```python
from build123d import *

# Parameters (mm, degrees)
SKETCH1_R           = 12.09
SKETCH1_R_2         = 1.75
SKETCH1_R_3         = 1.995
BOSS_EXTRUDE1_DEPTH = 4


with BuildPart() as part:
    # Sketch1 → Boss-Extrude1 (new body)
    # profile 1 of 22: a face of its own
    with BuildSketch(Plane.XY):
        Circle(SKETCH1_R)
        Circle(SKETCH1_R_2, mode=Mode.SUBTRACT)
    # profile 2 of 22: a face of its own
    with BuildSketch(Plane.XY):
        with BuildLine():
            ThreePointArc((14.051469909, -4.073462091), (14.048317136, -4.084321933), (14.04515597, -4.095179336))
            Line((14.04515597, -4.095179336), (30.82582707, -3.999919373))
            ThreePointArc((30.82582707, -3.999919373), (34.803112279, -0.008027822), (30.841914591, 3.999828048))
            Line((30.841914591, 3.999828048), (14.04515597, 4.095179336))
            ThreePointArc((14.04515597, 4.095179336), (14.128586435, 3.797360314), (14.205702589, 3.497844187))
            ThreePointArc((14.205702589, 3.497844187), (14.50484412, 1.909554151), (14.626965513, 0.297959519))
            ThreePointArc((14.626965513, 0.297959519), (14.629241359, 0.148987485), (14.63, 0))
            ThreePointArc((14.63, 0), (14.629241116, -0.149011314), (14.626964543, -0.298007168))
            ThreePointArc((14.626964543, -0.298007168), (14.504858624, -1.909443973), (14.20576712, -3.497582099))
            ThreePointArc((14.20576712, -3.497582099), (14.131552306, -3.786308154), (14.051469909, -4.073462091))
        make_face()
        with Locations((30.75, 0)):
            Circle(SKETCH1_R_3, mode=Mode.SUBTRACT)
    # profile 3 of 22: a face of its own
    with BuildSketch(Plane.XY):
        with BuildLine():
            ThreePointArc((14.205702589, 3.497844187), (14.128586435, 3.797360314), (14.04515597, 4.095179336))
            Line((14.04515597, 4.095179336), (13.966164937, 4.095627749))
            Line((13.966164937, 4.095627749), (11.369827915, 4.11036655))
            ThreePointArc((11.369827915, 4.11036655), (11.678097516, 3.128919686), (11.901816808, 2.124819208))
            ThreePointArc((11.901816808, 2.124819208), (13.1403578, 2.666023245), (14.205702589, 3.497844187))
        make_face()
    # profile 4 of 22: a face of its own
    with BuildSketch(Plane.XY):
        with BuildLine():
            ThreePointArc((-12.517636695, -7.572692492), (-11.175984377, -7.407777173), (-9.917325106, -6.914821961))
            ThreePointArc((-9.917325106, -6.914821961), (-10.469253219, -6.046721181), (-10.945386333, -5.134843524))
            ThreePointArc((-10.945386333, -5.134843524), (-12.001489862, -5.978375477), (-12.815033037, -7.057749518))
            ThreePointArc((-12.815033037, -7.057749518), (-12.668951436, -7.31673216), (-12.517636695, -7.572692492))
        make_face()
    # profile 5 of 22: a face of its own
    with BuildSketch(Plane.XY):
        with BuildLine():
            ThreePointArc((-14.051145033, -4.074582586), (-12.712516328, -4.262616236), (-11.369129658, -4.112297512))
            ThreePointArc((-11.369129658, -4.112297512), (-11.677558471, -3.130930876), (-11.901445615, -2.126897335))
            ThreePointArc((-11.901445615, -2.126897335), (-13.139881298, -2.668425004), (-14.205038564, -3.500539874))
            ThreePointArc((-14.205038564, -3.500539874), (-14.13100701, -3.788342761), (-14.051145033, -4.074582586))
        make_face()
    # profile 6 of 22: a face of its own
    with BuildSketch(Plane.XY):
        with BuildLine():
            ThreePointArc((-14.626950262, -0.298707293), (-13.382615157, -0.826868574), (-12.046093246, -1.029435529))
            ThreePointArc((-12.046093246, -1.029435529), (-12.089999882, -0.001686428), (-12.046379968, 1.026074882))
            ThreePointArc((-12.046379968, 1.026074882), (-13.382791491, 0.823465153), (-14.62701917, 0.295313712))
            ThreePointArc((-14.62701917, 0.295313712), (-14.629999902, -0.00169714), (-14.626950262, -0.298707293))
        make_face()
    # profile 7 of 22: a face of its own
    with BuildSketch(Plane.XY):
        with BuildLine():
            ThreePointArc((-14.205774364, 3.497552675), (-13.140565234, 2.66528054), (-11.902026335, 2.123645243))
            ThreePointArc((-11.902026335, 2.123645243), (-11.678416405, 3.127729251), (-11.370260409, 4.109170017))
            ThreePointArc((-11.370260409, 4.109170017), (-12.71360248, 4.259309779), (-14.052145793, 4.071129894))
            ThreePointArc((-14.052145793, 4.071129894), (-14.131870386, 3.78512079), (-14.205774364, 3.497552675))
        make_face()
    # profile 8 of 22: a face of its own
    with BuildSketch(Plane.XY):
        with BuildLine():
            ThreePointArc((-9.919135011, 6.912225448), (-11.177872267, 7.404913556), (-12.519533027, 7.569556974))
            ThreePointArc((-12.519533027, 7.569556974), (-12.670533379, 7.313992337), (-12.816317544, 7.055416686))
            ThreePointArc((-12.816317544, 7.055416686), (-12.00284137, 5.975783406), (-10.94671211, 5.132016561))
            ThreePointArc((-10.94671211, 5.132016561), (-10.470825179, 6.043998682), (-9.919135011, 6.912225448))
        make_face()
    # profile 9 of 22: a face of its own
    with BuildSketch(Plane.XY):
        with BuildLine():
            ThreePointArc((-7.791898403, 9.244155952), (-8.880242473, 10.045843984), (-10.13359017, 10.552120653))
            ThreePointArc((-10.13359017, 10.552120653), (-10.345575707, 10.344368676), (-10.553302948, 10.1323589))
            ThreePointArc((-10.553302948, 10.1323589), (-10.04699158, 8.878969486), (-9.245249077, 7.790601357))
            ThreePointArc((-9.245249077, 7.790601357), (-8.549520677, 8.54832125), (-7.791898403, 9.244155952))
        make_face()
    # profile 10 of 22: a face of its own
    with BuildSketch(Plane.XY):
        with BuildLine():
            ThreePointArc((-5.133551517, 10.945992364), (-5.977311447, 12.002061971), (-7.05691548, 12.815492339))
            ThreePointArc((-7.05691548, 12.815492339), (-7.315469666, 12.669680484), (-7.571012334, 12.518652972))
            ThreePointArc((-7.571012334, 12.518652972), (-7.40634855, 11.176941958), (-6.913615931, 9.918165897))
            ThreePointArc((-6.913615931, 9.918165897), (-6.045466706, 10.469977665), (-5.133551517, 10.945992364))
        make_face()
    # profile 11 of 22: a face of its own
    with BuildSketch(Plane.XY):
        with BuildLine():
            ThreePointArc((-2.125311093, 11.901728982), (-2.666957342, 13.14020836), (-3.499215334, 14.205364904))
            ThreePointArc((-3.499215334, 14.205364904), (-3.786765286, 14.131429817), (-4.072755654, 14.051674682))
            ThreePointArc((-4.072755654, 14.051674682), (-4.260931239, 12.713077321), (-4.110760617, 11.369685446))
            ThreePointArc((-4.110760617, 11.369685446), (-3.129363382, 11.677978627), (-2.125311093, 11.901728982))
        make_face()
    # profile 12 of 22: a face of its own
    with BuildSketch(Plane.XY):
        with BuildLine():
            ThreePointArc((1.027754616, 12.046236775), (0.825159863, 13.382704508), (0.296996585, 14.626985097))
            ThreePointArc((0.296996585, 14.626985097), (0, 14.63), (-0.296996585, 14.626985097))
            ThreePointArc((-0.296996585, 14.626985097), (-0.825159863, 13.382704508), (-1.027754616, 12.046236775))
            ThreePointArc((-1.027754616, 12.046236775), (0, 12.09), (1.027754616, 12.046236775))
        make_face()
    # profile 13 of 22: a face of its own
    with BuildSketch(Plane.XY):
        with BuildLine():
            ThreePointArc((4.110717434, 11.369701059), (4.260994095, 12.713043392), (4.072942889, 14.051620413))
            ThreePointArc((4.072942889, 14.051620413), (3.786710214, 14.131444574), (3.498915331, 14.2054388))
            ThreePointArc((3.498915331, 14.2054388), (2.666773966, 13.14023428), (2.125244746, 11.901740829))
            ThreePointArc((2.125244746, 11.901740829), (3.129308654, 11.677993293), (4.110717434, 11.369701059))
        make_face()
    # profile 14 of 22: a face of its own
    with BuildSketch(Plane.XY):
        with BuildLine():
            ThreePointArc((6.913450185, 9.91828143), (7.406352802, 11.176909529), (7.571236986, 12.518517105))
            ThreePointArc((7.571236986, 12.518517105), (7.315275528, 12.669792577), (7.056292749, 12.81583523))
            ThreePointArc((7.056292749, 12.81583523), (5.976880257, 12.002254067), (5.133331053, 10.946095756))
            ThreePointArc((5.133331053, 10.946095756), (6.045273784, 10.470089058), (6.913450185, 9.91828143))
        make_face()
    # profile 15 of 22: a face of its own
    with BuildSketch(Plane.XY):
        with BuildLine():
            ThreePointArc((9.244954117, 7.790951378), (10.046869152, 8.879052728), (10.553440202, 10.132215942))
            ThreePointArc((10.553440202, 10.132215942), (10.345229175, 10.344715236), (10.132740224, 10.552936821))
            ThreePointArc((10.132740224, 10.552936821), (8.879594749, 10.046380548), (7.791503622, 9.244488699))
            ThreePointArc((7.791503622, 9.244488699), (8.549176321, 8.548665641), (9.244954117, 7.790951378))
        make_face()
    # profile 16 of 22: a face of its own
    with BuildSketch(Plane.XY):
        with BuildLine():
            ThreePointArc((10.946374382, 5.132736881), (12.002615026, 5.976132183), (12.81632055, 7.055411226))
            ThreePointArc((12.81632055, 7.055411226), (12.670115094, 7.314716911), (12.518663963, 7.570994161))
            ThreePointArc((12.518663963, 7.570994161), (11.17714698, 7.405952739), (9.918639175, 6.912936924))
            ThreePointArc((9.918639175, 6.912936924), (10.47040953, 6.044718709), (10.946374382, 5.132736881))
        make_face()
    # profile 17 of 22: a face of its own
    with BuildSketch(Plane.XY):
        with BuildLine():
            ThreePointArc((12.046231207, -1.027819886), (11.986581537, -1.577961676), (11.901820644, -2.124797724))
            ThreePointArc((11.901820644, -2.124797724), (13.140374441, -2.665881604), (14.20576712, -3.497582099))
            ThreePointArc((14.20576712, -3.497582099), (14.504858624, -1.909443973), (14.626964543, -0.298007168))
            ThreePointArc((14.626964543, -0.298007168), (13.382627003, -0.825679814), (12.046231207, -1.027819886))
        make_face()
    # profile 18 of 22: a face of its own
    with BuildSketch(Plane.XY):
        with BuildLine():
            ThreePointArc((11.901820644, -2.124797724), (11.67810034, -3.128909147), (11.369827915, -4.11036655))
            Line((11.369827915, -4.11036655), (13.967019497, -4.095622898))
            ThreePointArc((13.967019497, -4.095622898), (14.009289492, -4.084713176), (14.051469909, -4.073462091))
            ThreePointArc((14.051469909, -4.073462091), (14.131552306, -3.786308154), (14.20576712, -3.497582099))
            ThreePointArc((14.20576712, -3.497582099), (13.140374441, -2.665881604), (11.901820644, -2.124797724))
        make_face()
    # profile 19 of 22: a face of its own
    with BuildSketch(Plane.XY):
        with BuildLine():
            ThreePointArc((12.09, 0), (12.079052845, -0.514375696), (12.046231207, -1.027819886))
            ThreePointArc((12.046231207, -1.027819886), (13.382627003, -0.825679814), (14.626964543, -0.298007168))
            ThreePointArc((14.626964543, -0.298007168), (14.629241116, -0.149011314), (14.63, 0))
            ThreePointArc((14.63, 0), (14.629241359, 0.148987485), (14.626965513, 0.297959519))
            ThreePointArc((14.626965513, 0.297959519), (13.382629481, 0.825632028), (12.046235232, 1.027772701))
            ThreePointArc((12.046235232, 1.027772701), (12.079053853, 0.514352039), (12.09, 0))
        make_face()
    # profile 20 of 22: a face of its own
    with BuildSketch(Plane.XY):
        with BuildLine():
            ThreePointArc((11.901816808, 2.124819208), (11.986583203, 1.577949019), (12.046235232, 1.027772701))
            ThreePointArc((12.046235232, 1.027772701), (13.382629481, 0.825632028), (14.626965513, 0.297959519))
            ThreePointArc((14.626965513, 0.297959519), (14.50484412, 1.909554151), (14.205702589, 3.497844187))
            ThreePointArc((14.205702589, 3.497844187), (13.1403578, 2.666023245), (11.901816808, 2.124819208))
        make_face()
    # profile 21 of 22: a face of its own
    with BuildSketch(Plane.XY):
        with BuildLine():
            Line((11.369827915, 4.11036655), (13.966164937, 4.095627749))
            ThreePointArc((13.966164937, 4.095627749), (12.668895431, 4.261362771), (11.369827915, 4.11036655))
        make_face()
    # profile 22 of 22: a face of its own
    with BuildSketch(Plane.XY):
        with BuildLine():
            ThreePointArc((-10.130994605, -10.554612656), (-8.877796666, -10.047999865), (-7.789679206, -9.246026058))
            ThreePointArc((-7.789679206, -9.246026058), (-8.547489799, -8.550351931), (-9.243417598, -7.792774288))
            ThreePointArc((-9.243417598, -7.792774288), (-10.045261463, -8.880834456), (-10.55179143, -10.133932978))
            ThreePointArc((-10.55179143, -10.133932978), (-10.343531911, -10.346412306), (-10.130994605, -10.554612656))
        make_face()
    extrude(amount=BOSS_EXTRUDE1_DEPTH)


solid = part.part
```
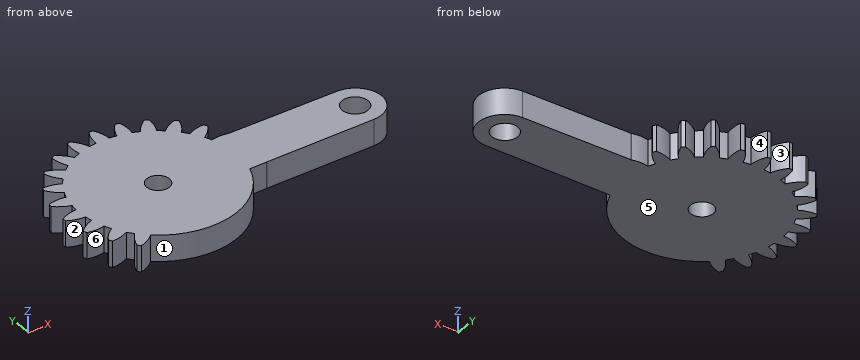
Here's how the part is built. I have some questions about the finished solid (model axes, mm). Face numbers are marked on the shaded views. A direction names the side the tool comes from. Round coordinates to 2 decimals unless told otherwise and drop trailing zeros. Order: outer loops, then holes, each group sorted by start corner. A loop starts at its lowest first (then second) coordinate and runs counter-clockwise, first axis right, second up. Notation, with made-up numbers: (81.25, -26.75) -> (111.25, -26.75) arc R21 cw to (111.25, -7.75) -> close; hole circle Ø10 at (57, 41). An arc over 180 degrees is marked (long way). Use a Markdown table: item, result. Add a question column.
(1) Suppose I cut it at B-B, the plane y = -8.75. Please give me the cut outline in (x, z).
(2) Suppose I cut it at A-A, the plane z = 2.65. Count the separate pieces of the cut face and the enclosed holes in it, and give its area (3 significant figures).
(3) Suppose I cut it at C-C, the plane x = 15.5. Please give me the cut outline in (y, z), and give its area (3 significant figures).
(4) For pin 1 Ø4 at (x, y) = (-4.5, -1) entering from -Z; pin 2 Ø3 at (x, y) = (30.75, 0) entering from -Z; pin 3 Ø1 at (x, z) = (-3, 3) entering from -Y, each with a flat end and sliding along its axis, tell me the tip position at first contact or that it passes through.
(5) For the marked faces 4, 5 and 6, which set-ups out of +Z, -Z, +X, -X, +Y, -Y let a thin tool reach every point of the face, with its end or its side?
(6) I need wall thicknesses on line 1 along Y through (x, z) = (0, 1.05); line 2 along Y through (x, z) = (30.75, 2.45) (3 decimals); line 3 along X through (y, z) = (10, 1.35). Which ranges of each line are inside material? Lowest first, please.
(7) If we mould it in two halves opening along Y, with no side actions, what happens to the marked faces 1, 2 and 3? For each: released by +Y, released by -Y, zero draft, split by the parting line, or undercut.
Verdict:
| question | item | result |
|---|---|---|
| 1 | outline | (-9.97, 0) -> (8.34, 0) -> (8.34, 4) -> (-9.97, 4) -> close |
| 2 | separate pieces | 1 |
| 2 | enclosed holes | 2 |
| 2 | area | 672 mm2 |
| 3 | outline | (-4.09, 0) -> (4.09, 0) -> (4.09, 4) -> (-4.09, 4) -> close |
| 3 | area | 32.7 mm2 |
| 4 | pin 1 | z = 0 |
| 4 | pin 2 | through |
| 4 | pin 3 | y = -11.83 |
| 5 | face 4 | +Z, -Z, +Y |
| 5 | face 5 | -Z, +X, -X, +Y, -Y |
| 5 | face 6 | +Z, -Z |
| 6 | line 1 | -12.09 to -1.75, 1.75 to 14.63 |
| 6 | line 2 | -4 to -1.995, 1.995 to 4 |
| 6 | line 3 | -10.52 to -8.8, -6.96 to 6.96, 8.8 to 10.52 |
| 7 | face 1 | released by -Y |
| 7 | face 2 | undercut |
| 7 | face 3 | released by +Y |
